Source: CAD feature listing. Evaluate the final solid. Frame: model axes, mm. Face numbers are marked on the shaded views. Round coordinates to 2 decimals unless told otherwise and drop trailing zeros. Order: outer loops, then holes, each group sorted by start corner. A loop starts at its lowest first (then second) coordinate and runs counter-clockwise, first axis right, second up. Notation, with made-up numbers: (-9, 42) -> (29, 42) arc R7 cw to (29, 50) -> close; hole circle Ø9 at (-7, -39.5). An arc over 180 degrees is marked (long way). One line per item, written item: value. Start each with the question number.
1) Section B-B (z = 0). Return the cut outline in (x, y).
2) Ray query, L1, parallel to Z at x = 0, y = 26; L2, parallel to X at y = 61.5, z = -20. Return the intervals inside material, ascending.
3) Mould query, pull axis X, two halves, no side actions, for the marked faces 1 and 2. Classes: pulls with the +X half, pulls with the -X half, needs draft (parallel to the pull), parting line crosses it, or undercut.
4) Pin query (flat end, axial travel): P1, Ø4, axis at y = 69, z = 9, coming from the -X side; P2, Ø3, axis at y = -97.5, z = 15, coming from the -X side; P3, Ø4, axis at x = -17, z = 12.5, coming from the -Y side; P4, Ø0.8, axis at x = 24.5, z = -2.5, coming from the -Y side. Return the tip coordinate at first contact, or that it passes through.
5) Section C-C (y = 48). Return the cut outline in (x, z).
6) Section A-A (x = 0). Return the cut outline in (y, z).
```python
from build123d import *

# Parameters (mm, degrees)
SKETCH1_R           = 25.4
SKETCH1_R_2         = 23.4
BOSS_EXTRUDE1_DEPTH = 125
CUT_EXTRUDE1_DEPTH  = 60


with BuildPart() as part:
    # Sketch1 → Boss-Extrude1 (new body, symmetric)
    with BuildSketch(Plane(origin=(0, 0, 0), x_dir=(1, 0, 0), z_dir=(0, 1, 0))):
        Circle(SKETCH1_R)
        Circle(SKETCH1_R_2, mode=Mode.SUBTRACT)
    extrude(amount=BOSS_EXTRUDE1_DEPTH, both=True)

    # Sketch2 → Cut-Extrude1 (cut)
    with BuildSketch(Plane.XZ.offset(125)):
        with BuildLine():
            Line((-24.719681161, -5.839294762), (-22.773249573, -5.379507773))
            ThreePointArc((-22.773249573, -5.379507773), (-23.4, 0), (-22.773249573, 5.379507773))
            Line((-22.773249573, 5.379507773), (-24.719681161, 5.839294762))
            ThreePointArc((-24.719681161, 5.839294762), (-25.4, 0), (-24.719681161, -5.839294762))
        make_face()
        with BuildLine():
            Line((24.719681161, -5.839294762), (22.773249573, -5.379507773))
            ThreePointArc((22.773249573, -5.379507773), (23.4, 0), (22.773249573, 5.379507773))
            Line((22.773249573, 5.379507773), (24.719681161, 5.839294762))
            ThreePointArc((24.719681161, 5.839294762), (25.4, 0), (24.719681161, -5.839294762))
        make_face()
    extrude(amount=-CUT_EXTRUDE1_DEPTH, mode=Mode.SUBTRACT)


solid = part.part
```
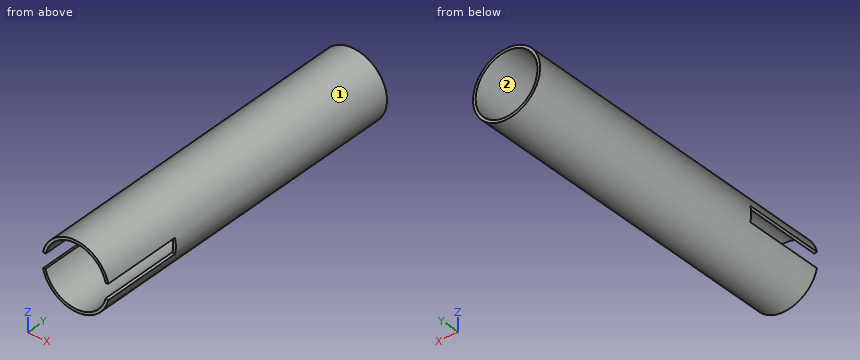
Findings:
1. outline: (-25.4, -65) -> (-23.4, -65) -> (-23.4, 125) -> (-25.4, 125) -> close; (23.4, -65) -> (25.4, -65) -> (25.4, 125) -> (23.4, 125) -> close
2. L1: -25.4 to -23.4, 23.4 to 25.4
2. L2: -15.66 to -12.15, 12.15 to 15.66
3. face 1: parting line crosses it
3. face 2: undercut
4. P1: x = -24.42
4. P2: x = -21.52
4. P3: through
4. P4: y = -65
5. outline: circle Ø50.8 at (0, 0); hole circle Ø46.8 at (0, 0)
6. outline: (-125, -25.4) -> (125, -25.4) -> (125, -23.4) -> (-125, -23.4) -> close; (-125, 23.4) -> (125, 23.4) -> (125, 25.4) -> (-125, 25.4) -> close
